Can you work these out from the model? Positions are in its coordinate system, mm. A direction names the side the tool comes from. Give positions to 0.01 mm unless a question says otherwise; leave off trailing zeros. Order: outer loops, then holes, each group sorted by start corner. A loop starts at its lowest first (then second) coordinate and runs counter-clockwise, first axis right, second up. Notation, with made-up numbers: (55, 78) - (79, 78) arc R36 ccw to (79, 117) - close; hole circle Ø6 at (48, 27.5). An arc over 180 degrees is marked (long way). Return JSON: item names as keys, results as strings.
```python
from build123d import *

# Parameters (mm, degrees)
F0_W          = 10.795
F0_H          = 131.347498
F1_DEPTH      = 127
F1_DEPTH_BACK = 127
F2_W          = 131.347498
F2_H          = 10.795
F3_DEPTH      = 254
F4_W          = 10.795
F4_H          = 131.347498
F5_DEPTH      = 254
F6_W          = 131.347498
F6_H          = 10.795
F7_DEPTH      = 254
F8_W          = 7.69969
F8_H          = 264.795
F9_DEPTH      = 254
F11_DEPTH     = 264.795


with BuildPart() as f1:
    # F0 (on Top) → F1 (new body, two sides)
    with BuildSketch(Plane.XY) as f1_sk:
        Rectangle(F0_W, F0_H)
    extrude(amount=F1_DEPTH)
    extrude(f1_sk.sketch, amount=-F1_DEPTH_BACK)

    # F2 (on face) → F3 (join)
    with BuildSketch(Plane.YZ.offset(5.3975)):
        with Locations((0, 121.6025)):
            Rectangle(F2_W, F2_H)
    extrude(amount=F3_DEPTH)

    # F4 (on face) → F5 (join)
    with BuildSketch(Plane(origin=(0, 0, 116.205), x_dir=(1, 0, 0), z_dir=(0, 0, -1))):
        with Locations((254, 0)):
            Rectangle(F4_W, F4_H)
    extrude(amount=F5_DEPTH)

    # F6 (on face) → F7 (join)
    with BuildSketch(Plane(origin=(248.6025, 0, 0), x_dir=(0, -1, 0), z_dir=(-1, 0, 0))):
        with Locations((0, -132.3975)):
            Rectangle(F6_W, F6_H)
    extrude(amount=F7_DEPTH)

    # F8 (on face) → F9 (join)
    with BuildSketch(Plane.YZ.offset(259.3975)):
        with Locations((-61.823904, -5.3975)):
            Rectangle(F8_W, F8_H)
    extrude(amount=-F9_DEPTH)

    # F10 (on face) → F11 (join)
    with BuildSketch(Plane(origin=(0, 0, -137.795), x_dir=(1, 0, 0), z_dir=(0, 0, -1))):
        Polygon((233.998537, -92.701845), (259.3975, -65.673749), (-5.3975, -65.673749), (30.545302, -99.291421), (138.861507, -162.71612), align=None)
    extrude(amount=-F11_DEPTH)


solid = f1.part
```
1. Suppose I cut it at C-C (z = 27.5). List the corners of the cut face in (x, y) for me.
Checks:
{"outline": "(-5.4, -65.67) - (259.4, -65.67) - (259.4, 65.67) - (234, 92.7) - (138.86, 162.72) - (30.55, 99.29) - (-5.4, 65.67) - close; hole (5.4, -57.97) - (248.6, -57.97) - (248.6, 65.67) - (5.4, 65.67) - close"}
2. Suppose I cut it at B-B (x = 146.5). List the corners of the cut face in (y, z) for me (3 decimals), plus the area to 3 significant figures.
Checks:
{"outline": "(-65.674, -137.795) - (157.095, -137.795) - (157.095, 127) - (-65.674, 127) - close; hole (-57.974, -127) - (65.674, -127) - (65.674, 116.205) - (-57.974, 116.205) - close", "area": "28,900 mm^2"}
3. If I drill on L1, parallel to Z at x = 47, y = 24.5 (3 decimals); L2, parallel to X at y = -2, z = 78; L3, parallel to Y at x = 115, z = -5, over which ranges is the centre line in solid material (lowest first)? Write a range as [from, to].
Checks:
{"L1": "[-137.795, -127], [116.205, 127]", "L2": "[-5.4, 5.4], [248.6, 259.4]", "L3": "[-65.67, -57.97], [65.67, 148.74]"}
4. On a 3-axis mill with a long thin cutter (end or side, diameter ignored), from which of +Z, -Z, +X, -X, +Y, -Y can I reach the whole of each face in a straight line? I mean faces 1 (the face through (12.322, 82.247, -7.251)), 2 (the face through (125, 3, 116.205)). Say none if no direction works.
Checks:
{"face 1": "+Z, -Z, -X, +Y", "face 2": "none"}
5. Suppose I cut it at D-D (y = 117). List the corners of the cut face in (x, z) for me (3 decimals).
Checks:
{"outline": "(60.788, -137.795) - (200.982, -137.795) - (200.982, 127) - (60.788, 127) - close"}
6. Thinking about a two-plate mould opening in X: for faces 3 (the face through (259.397, 1, -4)), 4 (the face through (-5.398, 1, -4)), 5 (the face through (129, -57.974, -7)), 6 (the face through (129, 65.674, -7)), which applies, +X half, -X half, draft (parallel to the pull), parting line (faces both ways), or undercut?
Checks:
{"face 3": "+X half", "face 4": "-X half", "face 5": "undercut", "face 6": "undercut"}
7. Suppose I cut it at A-A (y = 61.5). List the corners of the cut face in (x, z) for me (1 decimal).
Checks:
{"outline": "(-5.4, -137.8) - (259.4, -137.8) - (259.4, 127) - (-5.4, 127) - close; hole (5.4, -127) - (248.6, -127) - (248.6, 116.2) - (5.4, 116.2) - close"}
8. For pin 1 Ø5 at (y, z) = (96, 25) entering from +X; pin 2 Ø5 at (x, z) = (36.5, -39.5) entering from +Y; pin 3 Ø6 at (x, z) = (183.5, -106) entering from +Y, each with a flat end and sliding along its axis, tell me the tip position at first contact or that it passes through.
Checks:
{"pin 1": "x = 232.91", "pin 2": "y = 104.24", "pin 3": "y = 132.07"}
